Design review of the part built by this model. Coordinates are the model's own, in mm. A direction names the side the tool comes from. Coordinates: 2 decimals unless noted, no trailing zeros. Write each loop counter-clockwise with the first axis right and the second up, starting at its lowest first coordinate (ties: lowest second). Pieces come first, ordered by that corner, then holes. Notation, with made-up numbers: (72.25, -39) - (129.25, -39) arc R34 ccw to (129.25, -2) - close; hole circle Ø5 at (63, 0.25). An arc over 180 degrees is marked (long way). Answer as a JSON object with one key per item and string values.
```python
from build123d import *

# Parameters (mm, degrees)
SCHIZZO10_R                  = 20.675
ESTRUSIONE_ESTRUSIONE5_DEPTH = 43.2
TAGLIO_ESTRUSIONE11_DEPTH    = 23.1
FORO_25_5_25_4_1_D           = 25.4
FORO_25_5_25_4_1_DEPTH       = 17.6
FORO_25_5_25_4_1_CSINK_D     = 26
FORO_25_5_25_4_1_CSINK_ANGLE = 90
FORO_25_5_12_7_1_D           = 12.7
TAGLIO_ESTRUSIONE12_START    = -20.1
SCHIZZO24_R                  = 20.675
SCHIZZO24_R_2                = 10.668
TAGLIO_ESTRUSIONE12_DEPTH    = 20.1


with BuildPart() as part:
    # Schizzo10 → Estrusione-Estrusione5 (new body)
    with BuildSketch(Plane.XY):
        Circle(SCHIZZO10_R)
    extrude(amount=-ESTRUSIONE_ESTRUSIONE5_DEPTH)

    # Schizzo16 → Taglio-Estrusione11 (cut)
    with BuildSketch(Plane.XY):
        with BuildLine():
            Line((-17.905075223, 10.3375), (0, 20.675))
            ThreePointArc((0, 20.675), (-10.3375, 17.905075223), (-17.905075223, 10.3375))
        make_face()
        with BuildLine():
            ThreePointArc((17.905075223, 10.3375), (10.3375, 17.905075223), (0, 20.675))
            Line((0, 20.675), (17.905075223, 10.3375))
        make_face()
        with BuildLine():
            Line((-17.905075223, -10.3375), (-17.905075223, 10.3375))
            ThreePointArc((-17.905075223, 10.3375), (-20.675, 0), (-17.905075223, -10.3375))
        make_face()
        with BuildLine():
            Line((0, -20.675), (-17.905075223, -10.3375))
            ThreePointArc((-17.905075223, -10.3375), (-10.3375, -17.905075223), (0, -20.675))
        make_face()
        with BuildLine():
            ThreePointArc((0, -20.675), (10.3375, -17.905075223), (17.905075223, -10.3375))
            Line((17.905075223, -10.3375), (0, -20.675))
        make_face()
        with BuildLine():
            ThreePointArc((20.675, 0), (19.970516459, 5.351083757), (17.905075223, 10.3375))
            Line((17.905075223, 10.3375), (17.905075223, -10.3375))
            ThreePointArc((17.905075223, -10.3375), (19.970516459, -5.351083757), (20.675, 0))
        make_face()
    extrude(amount=-TAGLIO_ESTRUSIONE11_DEPTH, mode=Mode.SUBTRACT)

    # Foro Ø25.5 (25.4)-1
    with Locations(Plane.XY):
        with Locations((0, 0)):
            CounterSinkHole(FORO_25_5_25_4_1_D / 2, FORO_25_5_25_4_1_CSINK_D / 2, depth=FORO_25_5_25_4_1_DEPTH, counter_sink_angle=FORO_25_5_25_4_1_CSINK_ANGLE)

    # Foro Ø25.5 (12.7)-1 (through all)
    with Locations(Plane.XY.offset(-17.6)):
        with Locations((0, 0)):
            Hole(FORO_25_5_12_7_1_D / 2)

    # Schizzo24 → Taglio-Estrusione12 (cut)
    with BuildSketch(Plane(origin=(0, 0, -43.2), x_dir=(-1, 0, 0), z_dir=(0, 0, -1)).offset(TAGLIO_ESTRUSIONE12_START)):
        Circle(SCHIZZO24_R)
        Circle(SCHIZZO24_R_2, mode=Mode.SUBTRACT)
    extrude(amount=TAGLIO_ESTRUSIONE12_DEPTH, mode=Mode.SUBTRACT)


solid = part.part
```
(1) The part is to be moulded in two halves that separate along X. For faces 4 (the face through (9.078, -15.434, -11.388)), 5 (the face through (-0.3, -13.5, 0)), 6 (the face through (-8.827, -15.579, -11.388)), 7 (the face through (1.38, -6.2, -30.58)), say which applies: pulls with the +X half, pulls with the -X half, needs draft (parallel to the pull), parting line crosses it, or undercut.
Solved:
{"face 4": "pulls with the +X half", "face 5": "needs draft", "face 6": "pulls with the -X half", "face 7": "undercut"}
(2) Tool access review of faces 1 (the face through (-3, 6, -17.6)), 2 (the face through (8, -9, -23.1)), 3 (the face through (17.905, 0, -11)): name each direction out of +Z, -Z, +X, -X, +Y, -Y from which nothing blocks a thin tool from reaching the whole face with its end or side.
Solved:
{"face 1": "+Z", "face 2": "-Z", "face 3": "+Z, -Z, +X, +Y, -Y"}
(3) For pin 1 (1 mm diameter, centred on x = 3, z = -33.5, fed in from +Y); pin 2 (12 mm diameter, centred on y = 1.5, z = -37.5, fed in from -X); pin 3 (12.5 mm diameter, centred on x = 2, y = 4.5, fed in from +Z), all flat-tipped, find the tip position at first contact; note any pin that passes through.
Solved:
{"pin 1": "stops at y = 10.37", "pin 2": "stops at x = -10.67", "pin 3": "stops at z = -17.6"}
(4) To check wall thickness, follow line 1 (Y direction, x = 0, z = -29.5); line 2 (X direction, y = 0, z = -13.25); line 3 (Z direction, x = -5.5, y = -6.5). State the ranges of each line that lie inside material, in increasing order. Write a range as from..to.
Solved:
{"line 1": "y = -10.67..-6.35, 6.35..10.67", "line 2": "x = -17.91..-12.7, 12.7..17.91", "line 3": "z = -43.2..-17.6"}
(5) Take a section at B-B, the plane z = -14. Write out the cut boundary in (x, y) (1 decimal).
Solved:
{"outline": "(-17.9, -10.3) - (0, -20.7) - (17.9, -10.3) - (17.9, 10.3) - (0, 20.7) - (-17.9, 10.3) - close; hole circle Ø25.4 at (0, 0)"}
(6) Take a section at D-D, the plane x = -16. Write out the cut boundary in (y, z), and give its area (3 significant figures).
Solved:
{"outline": "(-11.44, -23.1) - (11.44, -23.1) - (11.44, 0) - (-11.44, 0) - close", "area": "528 mm^2"}
(7) Take a section at A-A, the plane y = 0. Write out the cut boundary in (x, z), and give its area (3 significant figures).
Solved:
{"outline": "(-17.91, -23.1) - (-10.67, -23.1) - (-10.67, -43.2) - (-6.35, -43.2) - (-6.35, -17.6) - (-12.7, -17.6) - (-12.7, -0.3) - (-13, 0) - (-17.91, 0) - close; (6.35, -43.2) - (10.67, -43.2) - (10.67, -23.1) - (17.91, -23.1) - (17.91, 0) - (13, 0) - (12.7, -0.3) - (12.7, -17.6) - (6.35, -17.6) - close", "area": "484 mm^2"}
